Source: CAD feature listing. Evaluate the final solid. Frame: model axes, mm. Face numbers are marked on the shaded views. A direction names the side the tool comes from. Coordinates: 2 decimals unless noted, no trailing zeros. Order: outer loops, then holes, each group sorted by start corner. A loop starts at its lowest first (then second) coordinate and runs counter-clockwise, first axis right, second up.
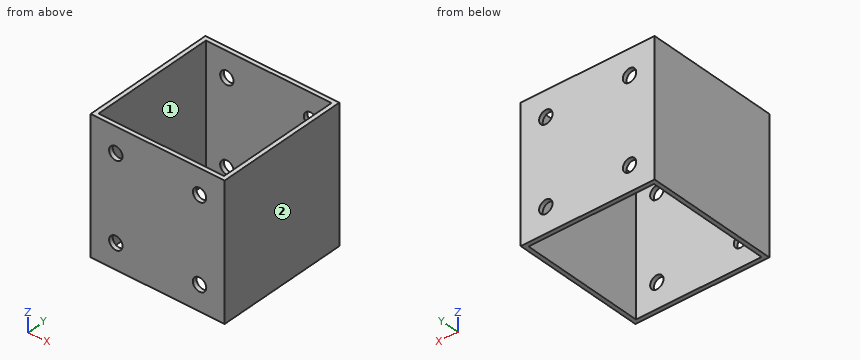
```python
from build123d import *

# Parameters (mm, degrees)
SKETCH2_W           = 50.8
SKETCH2_H           = 50.8
SKETCH2_W_2         = 47.625
SKETCH2_H_2         = 47.625
BOSS_EXTRUDE1_DEPTH = 50.8
SKETCH3_R           = 2.54
CUT_EXTRUDE1_DEPTH  = 88.988181024


with BuildPart() as part:
    # Sketch2 → Boss-Extrude1 (new body)
    with BuildSketch(Plane.XY):
        with Locations((25.4, 25.4)):
            Rectangle(SKETCH2_W, SKETCH2_H)
        with Locations((25.4, 25.4)):
            Rectangle(SKETCH2_W_2, SKETCH2_H_2, mode=Mode.SUBTRACT)
    extrude(amount=BOSS_EXTRUDE1_DEPTH)

    # Sketch3 → Cut-Extrude1 (cut, through all)
    with BuildSketch(Plane(origin=(0, 50.8, 0), x_dir=(1, 0, 0), z_dir=(0, 1, 0))):
        with Locations(Location((41.275, -9.525, 0), (0, 0, 270))):
            Circle(SKETCH3_R)
        with Locations(Location((41.275, -41.275, 0), (0, 0, 270))):
            Circle(SKETCH3_R)
        with Locations(Location((9.525, -9.525, 0), (0, 0, 270))):
            Circle(SKETCH3_R)
        with Locations(Location((9.525, -41.275, 0), (0, 0, 270))):
            Circle(SKETCH3_R)
    extrude(amount=-CUT_EXTRUDE1_DEPTH, mode=Mode.SUBTRACT)


solid = part.part
```
Q1. Set-up query: the marked faces 1 and 2. Return all of +Z, -Z, +X, -X, +Y, -Y with unobstructed straight access to the full face (end or side cutting, diameter ignored); none if empty.
Solutions:
face 1: +Z, -Z
face 2: +Z, -Z, +X, +Y, -Y
Q2. Section query C-C on z = 33. Output: boundary loops of the cut face in (x, y), plus the area to 4 significant figures.
Solutions:
outline: (0, 0) - (50.8, 0) - (50.8, 50.8) - (0, 50.8) - close; hole (1.59, 1.59) - (49.21, 1.59) - (49.21, 49.21) - (1.59, 49.21) - close
area: 312.5 mm2
Q3. Material intervals for line 1 along Y through (x, z) = (22, 8.5), sorted ascending.
Solutions:
line 1: y = 0 to 1.59, 49.21 to 50.8
Q4. Pin query (flat end, axial travel): P1, Ø4.5, axis at x = 41.275, z = 9.525, coming from the +Y side. Return the tip coordinate at first contact, or that it passes through.
Solutions:
P1: passes through
Q5. Section query A-A on x = 34. Output: boundary loops of the cut face in (y, z), plus the area to 3 significant figures.
Solutions:
outline: (0, 0) - (1.59, 0) - (1.59, 50.8) - (0, 50.8) - close; (49.21, 0) - (50.8, 0) - (50.8, 50.8) - (49.21, 50.8) - close
area: 161 mm2
Q6. Section query D-D on z = 42.5. Output: boundary loops of the cut face in (x, y).
Solutions:
outline: (0, 0) - (7.3, 0) - (7.3, 1.59) - (1.59, 1.59) - (1.59, 49.21) - (7.3, 49.21) - (7.3, 50.8) - (0, 50.8) - close; (11.75, 0) - (39.05, 0) - (39.05, 1.59) - (11.75, 1.59) - close; (11.75, 49.21) - (39.05, 49.21) - (39.05, 50.8) - (11.75, 50.8) - close; (43.5, 0) - (50.8, 0) - (50.8, 50.8) - (43.5, 50.8) - (43.5, 49.21) - (49.21, 49.21) - (49.21, 1.59) - (43.5, 1.59) - close
